Build history of the part. All positions in model axes, mm. Give positions to 0.01 mm unless a question says otherwise; leave off trailing zeros. Write each loop counter-clockwise with the first axis right and the second up, starting at its lowest first coordinate (ties: lowest second). Pieces come first, ordered by that corner, then holes.
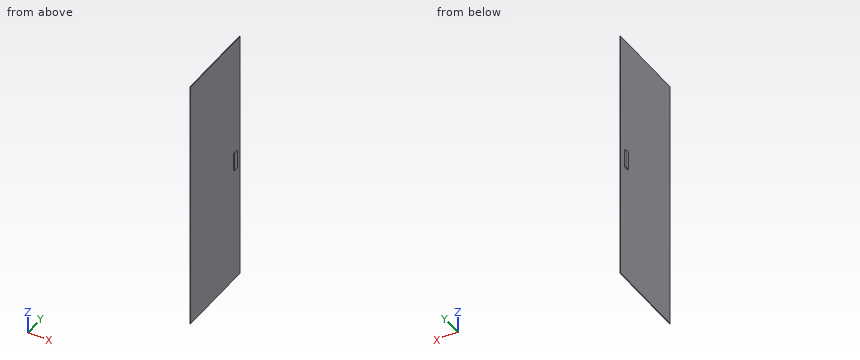
Autodesk Inventor part; units mm, degrees
ref_plane "YZ Plane" through (0, 0, 0) normal (1, 0, 0) x (0, 1, 0)
ref_plane "XZ Plane" through (0, 0, 0) normal (0, 1, 0) x (-1, 0, 0)
ref_plane "XY Plane" through (0, 0, 0) normal (0, 0, 1) x (1, 0, 0)
sketch "Sketch1" plane through (0, 0, 0) normal (1, 0, 0) x (0, 1, 0)
  line L0 (0, 0) -> (-363, 0)
  line L1 (-363, 0) -> (-363, 1118)
  line L2 (-363, 1118) -> (0, 1118)
  line L3 (0, 1118) -> (0, 0)
  dimension "d0" = 363
  dimension "d1" = 1118
extrude "Extrusion1" add sketch "Sketch1" against normal blind 3
sketch "Sketch2" plane through (0, 0, 0) normal (1, 0, 0) x (0, 0, -1)
  line L0 (-1118, 0) -> (-1118, -363)
  line L1 (-1118, -363) -> (0, -363)
  line L2 (0, -363) -> (0, 0)
  line L3 (0, 0) -> (-1118, 0)
  line L4 (-1118, 0) -> (0, 0) construction
  line L5 (-559, 0) -> (-559, -40) construction
  line L6 (-519, -30) -> (-599, -30)
  line L7 (-599, -30) -> (-599, -50)
  line L8 (-599, -50) -> (-519, -50)
  line L9 (-519, -50) -> (-519, -30)
  line L10 (-519, -30) -> (-599, -50) construction
  line L11 (-599, -30) -> (-519, -50) construction
  dimension "d4" = 40
  dimension "d5" = 80
  dimension "d6" = 20
extrude "Extrusion2" add sketch "Sketch2" along normal blind 6 and the other way blind 9 contours L9 L8 L7 L6
equation "\"d0\" = portaLargura"
properties part number "acrilicoMovel1"
1. Drill centre lines: line 1 along X through (y, z) = (-76, 536); line 2 along Z through (x, y) = (0.25, -46.5). Where is each one in solid material? Low to high.
2. Drop flat-ended pins along their axis: pin 1 (4 mm diameter, centred on y = -114, z = 229.5, fed in from +X); pin 2 (6.5 mm diameter, centred on x = -6.5, y = -38.5, fed in from -Z); pin 3 (5 mm diameter, centred on x = -6, z = 562, fed in from -Y). Give the stop position or say it passes through.
3. Saw through at B-B on y = -147. Give the cut face in (x, z), plus the area to 3 significant figures.
4. Saw through at A-A on x = -6. Give the cut face in (y, z).
Outcome:
1. line 1: x = -3 to 0
1. line 2: z = 519 to 599
2. pin 1: stops at x = 0
2. pin 2: stops at z = 519
2. pin 3: stops at y = -50
3. outline: (-3, 0) - (0, 0) - (0, 1118) - (-3, 1118) - close
3. area: 3,350 mm2
4. outline: (-50, 519) - (-30, 519) - (-30, 599) - (-50, 599) - close
